```python
from build123d import *

# Parameters (mm, degrees)
BOSS_EXTRUDE2_DEPTH         = 152.4
CUT_EXTRUDE1_DEPTH          = 157.576115675
SKETCH5_R                   = 3.3782
CUT_EXTRUDE2_DEPTH          = 157.576115675
CUT_EXTRUDE3_REACH          = 158.576
SKETCH10_R                  = 3.3782
F_1_4_CLEARANCE_HOLE1_D     = 6.7564
F_1_4_CLEARANCE_HOLE1_DEPTH = 25.4
F_1_4_CLEARANCE_HOLE1_TIP   = 2.029827343


with BuildPart() as part:
    # Sketch3 → Boss-Extrude2 (new, symmetric)
    with BuildSketch(Plane.XY):
        Polygon((-12.7, 25.4), (-12.7, -25.4), (12.7, -25.4), (12.7, 25.4), (9.525, 25.4), (9.525, -22.225), (-9.525, -22.225), (-9.525, 25.4), align=None)
    extrude(amount=BOSS_EXTRUDE2_DEPTH, both=True)

    # Sketch4 → Cut-Extrude1 (cut, through all)
    with BuildSketch(Plane(origin=(12.7, 0, 0), x_dir=(0, 0, -1), z_dir=(1, 0, 0))):
        Polygon((-152.4, 25.4), (-101.6, -25.4), (-152.4, -25.4), align=None)
    extrude(amount=-CUT_EXTRUDE1_DEPTH, mode=Mode.SUBTRACT)

    # Sketch5 → Cut-Extrude2 (cut, through all)
    with BuildSketch(Plane.ZY.offset(12.7)):
        with Locations(Location((-8.209871939, 8.209871939, 0), (0, 0, 270))):
            Circle(SKETCH5_R)
        with Locations(Location((-17.190128061, 17.190128061, 0), (0, 0, 270))):
            Circle(SKETCH5_R)
    extrude(amount=-CUT_EXTRUDE2_DEPTH, mode=Mode.SUBTRACT)

    # Cut-Extrude3: up to this face of the body (flat: up to its plane)
    cut_extrude3_end = Plane(part.part.faces().sort_by_distance((12.7, 0.709119442, -12.313197401))[0])
    # Sketch10 → Cut-Extrude3 (cut, up to the picked face)
    with BuildSketch(Plane.ZY.offset(12.7), mode=Mode.PRIVATE) as cut_extrude3_sk1:
        with Locations(Location((66.317182668, 12.7, 0), (0, 0, 270))):
            Circle(SKETCH10_R)
    cut_extrude3_tool1 = split(extrude(cut_extrude3_sk1.sketch, amount=-CUT_EXTRUDE3_REACH, mode=Mode.PRIVATE), bisect_by=cut_extrude3_end, keep=Keep.BOTH, mode=Mode.PRIVATE)
    # Sketch10 → Cut-Extrude3 (cut, up to the picked face)
    with BuildSketch(Plane.ZY.offset(12.7), mode=Mode.PRIVATE) as cut_extrude3_sk2:
        with Locations(Location((129.178975516, 12.7, 0), (0, 0, 270))):
            Circle(SKETCH10_R)
    cut_extrude3_tool2 = split(extrude(cut_extrude3_sk2.sketch, amount=-CUT_EXTRUDE3_REACH, mode=Mode.PRIVATE), bisect_by=cut_extrude3_end, keep=Keep.BOTH, mode=Mode.PRIVATE)
    # Sketch10 → Cut-Extrude3 (cut, up to the picked face)
    with BuildSketch(Plane.ZY.offset(12.7), mode=Mode.PRIVATE) as cut_extrude3_sk3:
        with Locations(Location((102.238207153, 12.7, 0), (0, 0, 270))):
            Circle(SKETCH10_R)
    cut_extrude3_tool3 = split(extrude(cut_extrude3_sk3.sketch, amount=-CUT_EXTRUDE3_REACH, mode=Mode.PRIVATE), bisect_by=cut_extrude3_end, keep=Keep.BOTH, mode=Mode.PRIVATE)
    add(cut_extrude3_tool1.solids().sort_by(Axis((-12.7, 12.7, 66.317183), (1, 0, 0)))[0], mode=Mode.SUBTRACT)
    add(cut_extrude3_tool2.solids().sort_by(Axis((-12.7, 12.7, 129.178976), (1, 0, 0)))[0], mode=Mode.SUBTRACT)
    add(cut_extrude3_tool3.solids().sort_by(Axis((-12.7, 12.7, 102.238207), (1, 0, 0)))[0], mode=Mode.SUBTRACT)

    # 1/4 Clearance Hole1
    with Locations(Plane.ZY.offset(12.7)):
        with Locations((38.1, -12.7), (-114.3, -12.7), (-76.2, -12.7)):
            Hole(F_1_4_CLEARANCE_HOLE1_D / 2, depth=F_1_4_CLEARANCE_HOLE1_DEPTH)
            with Locations((0, 0, -(F_1_4_CLEARANCE_HOLE1_DEPTH + F_1_4_CLEARANCE_HOLE1_TIP / 2))):  # 118° drill point
                Cone(0, F_1_4_CLEARANCE_HOLE1_D / 2, F_1_4_CLEARANCE_HOLE1_TIP, mode=Mode.SUBTRACT)


solid = part.part
```
Input: part model. Units: mm. Frame: model coordinates. A direction names the side the tool comes from. Coordinates: 2 decimals unless noted, no trailing zeros. Write each loop counter-clockwise with the first axis right and the second up, starting at its lowest first coordinate (ties: lowest second). Pieces come first, ordered by that corner, then holes. Notation, with made-up numbers: (-2.5, -25) -> (46.5, -25) arc R26 ccw to (46.5, -5) -> close; hole circle Ø2 at (76.25, 32.25). An arc over 180 degrees is marked (long way). Answer as a JSON object with one key per item and string values.
1. Section D-D on z = 37.5. Return the cut outline in (x, y) (1 decimal).
Result set:
{"outline": "(-12.7, -25.4) -> (12.7, -25.4) -> (12.7, -16) -> (9.5, -16) -> (9.5, -22.2) -> (-9.5, -22.2) -> (-9.5, -16) -> (-12.7, -16) -> close; (-12.7, -9.4) -> (-9.5, -9.4) -> (-9.5, 25.4) -> (-12.7, 25.4) -> close; (9.5, -9.4) -> (12.7, -9.4) -> (12.7, 25.4) -> (9.5, 25.4) -> close"}
2. Section B-B on y = -12.7. Count the separate pieces of the cut face and the enclosed holes in it, then the cut area to 3 significant figures.
Result set:
{"separate pieces": "8", "enclosed holes": "0", "area": "1,560 mm2"}
3. Mould query, pull axis X, two halves, no side actions, for faces 3 (the face through (-11.13, 13.43, 63.02)), 4 (the face through (0, -22.225, -22)), 5 (the face through (-9.525, 1, 2)). Classes: released by +X, released by -X, zero draft, split by the parting line, or undercut.
Result set:
{"face 3": "zero draft", "face 4": "undercut", "face 5": "undercut"}
4. Section A-A on z = -114.3. Return the cut outline in (x, y) (3 decimals), then the cut area to 3 significant figures.
Result set:
{"outline": "(-12.7, -25.4) -> (12.7, -25.4) -> (12.7, -16.078) -> (9.525, -16.078) -> (9.525, -22.225) -> (-9.525, -22.225) -> (-9.525, -16.078) -> (-12.7, -16.078) -> close; (-12.7, -9.322) -> (-9.525, -9.322) -> (-9.525, 25.4) -> (-12.7, 25.4) -> close; (9.525, -9.322) -> (12.7, -9.322) -> (12.7, 25.4) -> (9.525, 25.4) -> close", "area": "340 mm2"}
5. Access query for faces 1 (the face through (9.525, 2, 2)), 2 (the face through (11.09, 11.14, 99.24)). Directions: +Z, -Z, +X, -X, +Y, -Y. A direction counts if a zero-diameter tool reaches every point of the face in a straight line with its end or side. Return the directions, or none.
Result set:
{"face 1": "+Z, -Z, +Y", "face 2": "+X, -X"}
6. First-contact query: P1, Ø4, axis at x = 8, y = 8.5, coming from the +Z side; P2, Ø10, axis at x = -9, y = -14, coming from the +Z side; P3, Ø9.5, axis at x = 3.5, z = -1, coming from the +Y side (3 decimals). Flat tips, straight axial feed; report the tip coordinate or a pass-through.
Result set:
{"P1": "stops at z = 136.79", "P2": "stops at z = 117.97", "P3": "stops at y = -22.225"}
7. Section C-C on x = 0.25. Return the cut outline in (y, z) (3 decimals), then the cut area to 3 significant figures.
Result set:
{"outline": "(-25.4, -152.4) -> (-22.225, -152.4) -> (-22.225, 104.775) -> (-25.4, 101.6) -> close", "area": "811 mm2"}
8. Material intervals for line 1 (X direction, y = -19, z = -58) (3 decimals); line 2 (Y direction, x = -11.6, z = -76.2); line 3 (Z direction, x = -11.1, y = 12.7), sorted ascending. Write a range as from..to.
Result set:
{"line 1": "x = -12.7..-9.525, 9.525..12.7", "line 2": "y = -25.4..-16.08, -9.32..25.4", "line 3": "z = -152.4..62.94, 69.7..98.86, 105.62..125.8, 132.56..139.7"}
